from build123d import *

# Parameters (mm, degrees)
F2_SIZE  = 2.5
F3_R     = 6.5
F4_DEPTH = 45.501
F5_START = 18.5
F3_R_2   = 14.5
F5_DEPTH = 7
F6_SIZE  = 2.5


with BuildPart() as f1:
    # F0 (on Front) → F1 (revolve)
    with BuildSketch(Plane.XZ):
        Polygon((0, 84.45), (0, 45), (5, 45), (5, 10), (20.5, 10), (20.5, 5), (45.5, 5), (45.5, 25), (38.3, 25), (38.3, 14.5), (25.5, 14.5), (25.5, 84.45), (15.5, 84.45), (15.5, 79.45), (10, 79.45), (10, 84.45), align=None)
    revolve(axis=Axis((36.0234118998, 0, 0), (1, 0, 0)))

    # F2
    f2_edges = [f1.edges().sort_by_distance(p)[0] for p in [
        (25.5, 0, -84.45),
        (15.5, 0, -84.45),
        (10, 0, -84.45),
        (0, 0, -84.45),
    ]]
    chamfer(f2_edges, length=F2_SIZE)

    # F3 (on Right) → F4 (cut, through all)
    with BuildSketch(Plane.YZ):
        with Locations((57.0633909777, 18.5410196625)):
            Circle(F3_R)
        with Locations((35.2671151375, -48.5410196625)):
            Circle(F3_R)
        with Locations((-35.2671151375, -48.5410196625)):
            Circle(F3_R)
        with Locations((-57.0633909777, 18.5410196625)):
            Circle(F3_R)
        with Locations((0, 60)):
            Circle(F3_R)
    extrude(amount=F4_DEPTH, mode=Mode.SUBTRACT)

    # F3 (on Right) → F5 (cut)
    with BuildSketch(Plane.YZ.offset(F5_START)):
        with Locations((0, 60)):
            Circle(F3_R_2)
        with Locations((0, 60)):
            Circle(F3_R, mode=Mode.SUBTRACT)
        with Locations((-57.0633909777, 18.5410196625)):
            Circle(F3_R_2)
        with Locations((-57.0633909777, 18.5410196625)):
            Circle(F3_R, mode=Mode.SUBTRACT)
        with Locations((-35.2671151375, -48.5410196625)):
            Circle(F3_R_2)
        with Locations((-35.2671151375, -48.5410196625)):
            Circle(F3_R, mode=Mode.SUBTRACT)
        with Locations((35.2671151375, -48.5410196625)):
            Circle(F3_R_2)
        with Locations((35.2671151375, -48.5410196625)):
            Circle(F3_R, mode=Mode.SUBTRACT)
        with Locations((57.0633909777, 18.5410196625)):
            Circle(F3_R_2)
        with Locations((57.0633909777, 18.5410196625)):
            Circle(F3_R, mode=Mode.SUBTRACT)
    extrude(amount=F5_DEPTH, mode=Mode.SUBTRACT)

    # F6
    f6_edges = [f1.edges().sort_by_distance(p)[0] for p in [
        (45.5, 0, -25),
        (38.3, 0, -25),
    ]]
    chamfer(f6_edges, length=F6_SIZE)


solid = f1.part
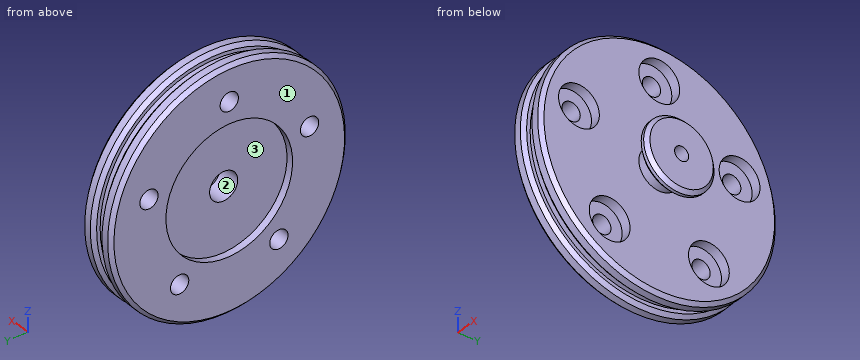
CAD build for the part. Positions are in the model's coordinates, mm. Face numbers are marked on the shaded views. Coordinates: 2 decimals unless noted, no trailing zeros. Write item = value, one per line. Start each with the question number.
Q1. Drill centre lines: L1, parallel to Z at x = 20.25, y = 0; L2, parallel to Z at x = 14, y = 0; L3, parallel to Y at x = 31.5, z = 0. Where is each one in solid material? Low to high.
Q2. Cut at A-A, the plane y = 0. Give the number of separate pieces and of enclosed holes in the cut face, then the cut area to 3 significant figures.
Q3. Pull direction Z, two halves, no side cores. Call the marked faces 1, 2 and 3: pulls with the +Z half, pulls with the -Z half, needs draft (parallel to the pull), parting line crosses it, or undercut.
Q4. Flat gauge pins, fed straight in: pin 1 Ø8.5 at (y, z) = (-6.5, 57.5) entering from +X; pin 2 Ø1.5 at (y, z) = (-3.5, -5) entering from -X; pin 3 Ø22 at (y, z) = (-2, 0.5) entering from -X; pin 4 Ø10.5 at (y, z) = (35.27, -48.54) entering from -X. Where does each tip first touch, or does it go through?
Computed:
q1.L1 = -84.45 to -10, 10 to 45.5, 74.5 to 84.45
q1.L2 = -79.45 to -10, 10 to 53.5, 66.5 to 79.45
q1.L3 = -14.5 to -5, 5 to 14.5
q2.separate_pieces = 3
q2.enclosed_holes = 0
q2.area = 3,490 mm²
q3.face_1 = needs draft
q3.face_2 = undercut
q3.face_3 = undercut
q4.pin_1 = 18.5
q4.pin_2 = 20.5
q4.pin_3 = 5
q4.pin_4 = through
